The model under review builds one solid part; all positions refer to its coordinate system, in mm. Round coordinates to 2 decimals unless told otherwise and drop trailing zeros. Order: outer loops, then holes, each group sorted by start corner. A loop starts at its lowest first (then second) coordinate and runs counter-clockwise, first axis right, second up. Notation, with made-up numbers: M 74,34 L 106,34 A31 ccw 106,65 Z; hole C 74.25,-7 d5. An arc over 180 degrees is marked long. Answer as a JSON object with one key per item and string values. Group by question number.
1. To check wall thickness, follow probe 1 along X at (y, z) = (-1.25, 0); probe 2 along X at (y, z) = (-1.2, 2). State the ranges of each line that lie inside material, in increasing order. Write a range as [from, to].
2. Add section A-A on z = 0. State the section outline as (x, y) points, and give its area (3 significant figures).
3. Add section B-B on x = 70. State the section outline as (y, z) points, and give its area (3 significant figures).
4. Mouldability with a two-part tool opening along X and no side actions: class faces 1 (the face through (1, 0, 0)), 2 (the face through (-67.52, -0.99, -0.33)) as released by +X, released by -X, zero draft, split by the parting line, or undercut.
```python
from build123d import *

# Parameters (mm, degrees)
SKETCH_1_R             = 2.5
SM_BASE_FLANGE_1_DEPTH = 2


# Sheet-metal steps are written as plain solids
with BuildPart() as part:
    # Sketch 1 → 基体-法兰1 (new body)
    with BuildSketch(Plane(origin=(0, 0, 0), x_dir=(1, 0, 0), z_dir=(0, 1, 0))):
        with BuildLine():
            Line((-78, 10), (78, 10))
            ThreePointArc((78, 10), (79.414213562, 9.414213562), (80, 8))
            Line((80, 8), (80, -8))
            ThreePointArc((80, -8), (79.414213562, -9.414213562), (78, -10))
            Line((78, -10), (-78, -10))
            ThreePointArc((-78, -10), (-79.414213562, -9.414213562), (-80, -8))
            Line((-80, -8), (-80, 8))
            ThreePointArc((-80, 8), (-79.414213562, 9.414213562), (-78, 10))
        make_face()
        with Locations(Location((-70, 0, 0), (0, 0, 270))):
            Circle(SKETCH_1_R, mode=Mode.SUBTRACT)
        with Locations(Location((70, 0, 0), (0, 0, 270))):
            Circle(SKETCH_1_R, mode=Mode.SUBTRACT)
    extrude(amount=-SM_BASE_FLANGE_1_DEPTH)


solid = part.part
```
Recorded:
{
 "1": {"probe 1": "x = [-80, -72.5], [-67.5, 67.5], [72.5, 80]", "probe 2": "x = [-80, -71.5], [-68.5, 68.5], [71.5, 80]"},
 "2": {"outline": "M -80,-2 L -72.5,-2 L -72.5,0 L -80,0 Z; M -67.5,-2 L 67.5,-2 L 67.5,0 L -67.5,0 Z; M 72.5,-2 L 80,-2 L 80,0 L 72.5,0 Z", "area": "300 mm²"},
 "3": {"outline": "M -2,-10 L 0,-10 L 0,-2.5 L -2,-2.5 Z; M -2,2.5 L 0,2.5 L 0,10 L -2,10 Z", "area": "30.0 mm²"},
 "4": {"face 1": "zero draft", "face 2": "undercut"}
}
